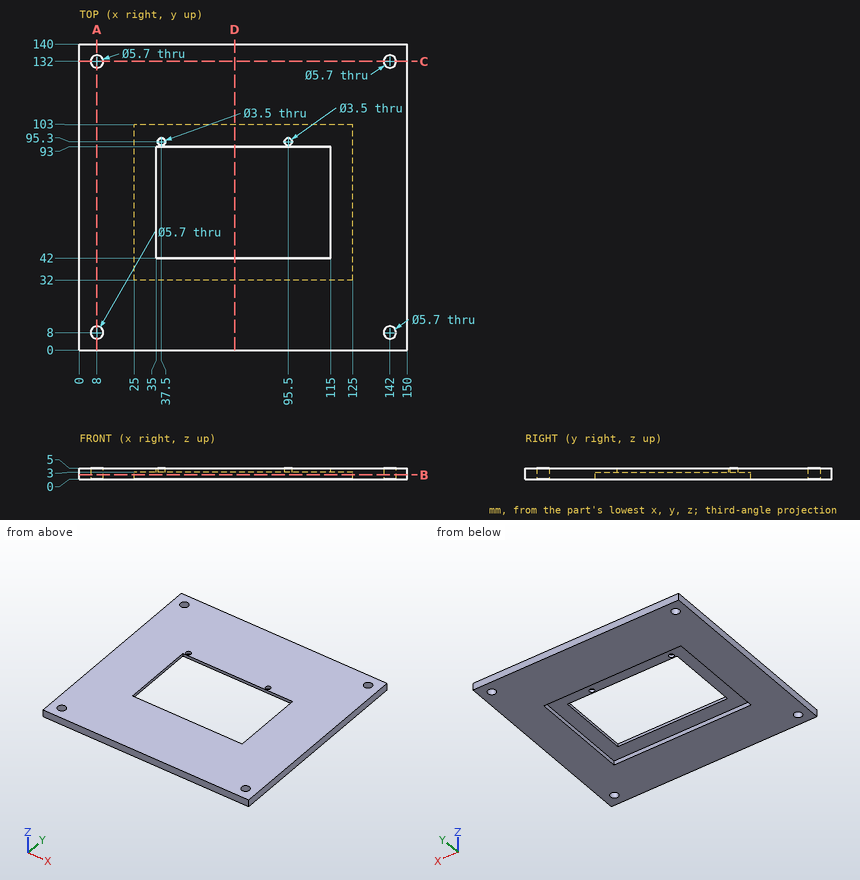
Source: three-view drawing plus pictorial views. Frame: mm from the lowest corner of the part. Round coordinates to 2 decimals unless told otherwise and drop trailing zeros. Loops run counter-clockwise (first coordinate to the right, second up) from the corner with the lowest first, then second, coordinate; pieces in that order, holes last. Notation, with made-up numbers: M 32.25,-14.75 L 79.25,-14.75 A21 cw 79.25,3.25 Z; hole C 77.5,65 d3. An arc over 180 degrees is marked long. Put each result on its own line as item: value.
(1) Section D-D, the plane x = 71. Return loops of the section in (y, z), and give its area (3 significant figures).
Solutions:
outline: M 0,0 L 32,0 L 32,3 L 42,3 L 42,5 L 0,5 Z; M 93,3 L 103,3 L 103,0 L 140,0 L 140,5 L 93,5 Z
area: 385 mm²
(2) Section A-A, the plane x = 8. Return loops of the section in (y, z).
Solutions:
outline: M 0,0 L 5.15,0 L 5.15,5 L 0,5 Z; M 10.85,0 L 129.15,0 L 129.15,5 L 10.85,5 Z; M 134.85,0 L 140,0 L 140,5 L 134.85,5 Z
(3) Ray query, line 1 (X direction, y = 95.3, z = 4.15); line 2 (X direction, y = 132, z = 1.05); line 3 (Y direction, x = 37.5, z = 3.95). Return the intervals inside material, ascending. Write a range as [from, to].
Solutions:
line 1: [0, 35.75], [39.25, 93.75], [97.25, 150]
line 2: [0, 5.15], [10.85, 139.15], [144.85, 150]
line 3: [0, 42], [93, 93.55], [97.05, 140]
(4) Section C-C, the plane y = 132. Return loops of the section in (x, z).
Solutions:
outline: M 0,0 L 5.15,0 L 5.15,5 L 0,5 Z; M 10.85,0 L 139.15,0 L 139.15,5 L 10.85,5 Z; M 144.85,0 L 150,0 L 150,5 L 144.85,5 Z
(5) First-contact query: pin 1 (1.5 mm diameter, centred on x = 90.5, y = 92, fed in from +Z); pin 2 (4.5 mm diameter, centred on x = 95.5, y = 95.3, fed in from +Z); pin 3 (4 mm diameter, centred on x = 37.5, y = 95.3, fed in from -Z). Flat tips, straight axial feed; report the tip coordinate or a pass-through.
Solutions:
pin 1: through
pin 2: z = 5
pin 3: z = 3
(6) Section B-B, the plane z = 1.9. Return loops of the section in (x, y), and give its area (3 significant figures).
Solutions:
outline: M 0,0 L 150,0 L 150,140 L 0,140 Z; hole C 8,8 d5.7; hole C 8,132 d5.7; hole M 25,32 L 125,32 L 125,103 L 25,103 Z; hole C 142,8 d5.7; hole C 142,132 d5.7
area: 13,800 mm²
